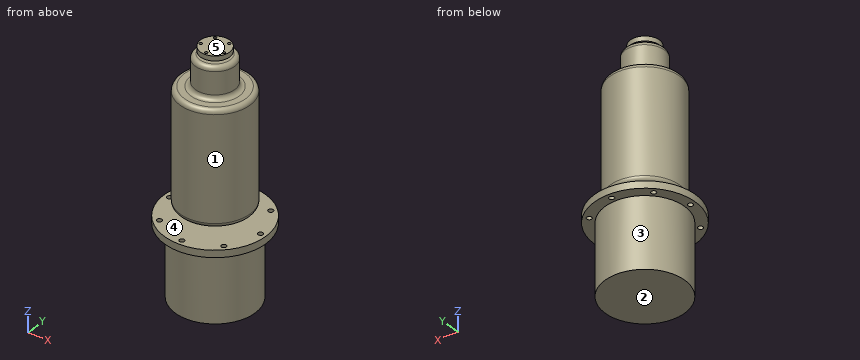
from build123d import *

# Parameters (mm, degrees)
SKETCH1_R          = 57.15
EXTRUDE1_DEPTH     = 4
SKETCH3_R          = 7.5
EXTRUDE2_DEPTH     = 12.166
SKETCH4_R          = 39.5
EXTRUDE3_DEPTH     = 127.24
SKETCH5_R          = 22.225
EXTRUDE4_DEPTH     = 35.083496
SKETCH6_R          = 9.525
EXTRUDE5_DEPTH     = 2.702052
SKETCH7_R          = 16.5
EXTRUDE6_DEPTH     = 5.3848
SKETCH8_R          = 1.6
CUT_EXTRUDE1_DEPTH = 5.3848
SKETCH10_R         = 2.79
CUT_EXTRUDE2_DEPTH = 8
SKETCH11_R         = 45
EXTRUDE7_DEPTH     = 79.4
FILLET1_R          = 5


with BuildPart() as part:
    # Sketch1 → Extrude1 (new body, symmetric)
    with BuildSketch(Plane.XY):
        Circle(SKETCH1_R)
    extrude(amount=EXTRUDE1_DEPTH, both=True)

    # Sketch3 → Extrude2 (add)
    with BuildSketch(Plane.XY.offset(4)):
        Circle(SKETCH3_R)
    extrude(amount=EXTRUDE2_DEPTH)

    # Sketch4 → Extrude3 (add)
    with BuildSketch(Plane.XY.offset(16.166)):
        Circle(SKETCH4_R)
    extrude(amount=EXTRUDE3_DEPTH)

    # Sketch5 → Extrude4 (add)
    with BuildSketch(Plane.XY.offset(143.406)):
        Circle(SKETCH5_R)
    extrude(amount=EXTRUDE4_DEPTH)

    # Sketch6 → Extrude5 (add)
    with BuildSketch(Plane.XY.offset(178.489496)):
        Circle(SKETCH6_R)
    extrude(amount=EXTRUDE5_DEPTH)

    # Sketch7 → Extrude6 (add)
    with BuildSketch(Plane.XY.offset(181.191548)):
        Circle(SKETCH7_R)
    extrude(amount=EXTRUDE6_DEPTH)

    # Sketch8 → Cut-Extrude1 (cut)
    with BuildSketch(Plane.XY.offset(186.576348)):
        with Locations((-7.935100906, 10.921729424)):
            Circle(SKETCH8_R)
        with Locations((7.935100906, 10.921729424)):
            Circle(SKETCH8_R)
        with Locations((12.83926297, -4.171729424)):
            Circle(SKETCH8_R)
        with Locations((0, -13.5)):
            Circle(SKETCH8_R)
        with Locations((-12.83926297, -4.171729424)):
            Circle(SKETCH8_R)
    extrude(amount=-CUT_EXTRUDE1_DEPTH, mode=Mode.SUBTRACT)

    # Sketch10 → Cut-Extrude2 (cut)
    with BuildSketch(Plane(origin=(0, 0, -4), x_dir=(-1, 0, 0), z_dir=(0, 0, -1))):
        with Locations((0, 50.8)):
            Circle(SKETCH10_R)
        with Locations((35.921024484, 35.921024484)):
            Circle(SKETCH10_R)
        with Locations((50.8, 0)):
            Circle(SKETCH10_R)
        with Locations((35.921024484, -35.921024484)):
            Circle(SKETCH10_R)
        with Locations((0, -50.8)):
            Circle(SKETCH10_R)
        with Locations((-35.921024484, -35.921024484)):
            Circle(SKETCH10_R)
        with Locations((-50.8, 0)):
            Circle(SKETCH10_R)
        with Locations((-35.921024484, 35.921024484)):
            Circle(SKETCH10_R)
    extrude(amount=-CUT_EXTRUDE2_DEPTH, mode=Mode.SUBTRACT)

    # Sketch11 → Extrude7 (add)
    with BuildSketch(Plane(origin=(0, 0, -4), x_dir=(-1, 0, 0), z_dir=(0, 0, -1))):
        with Locations(Location((0, 0, 0), (0, 0, 180))):  # turned: the seam where the file's is
            Circle(SKETCH11_R)
    extrude(amount=EXTRUDE7_DEPTH)

    # Fillet1
    fillet1_edges = [part.edges().sort_by_distance(p)[0] for p in [
        (-39.5, 0, 143.406),
        (-22.225, 0, 143.406),
        (-22.225, 0, 178.489496),
        (-39.5, 0, 16.166),
    ]]
    fillet(fillet1_edges, radius=FILLET1_R)


solid = part.part
The listing builds one solid part. Answer for the finished solid, in the listing's coordinates (mm). Face numbers are marked on the shaded views. A direction names the side the tool comes from. Round coordinates to 2 decimals unless told otherwise and drop trailing zeros. Write each loop counter-clockwise with the first axis right and the second up, starting at its lowest first coordinate (ties: lowest second). Pieces come first, ordered by that corner, then holes. Notation, with made-up numbers: (-34.5, 61) - (-27.5, 61) arc R23 cw to (-27.5, 74) - close; hole circle Ø11 at (-11.5, 84). An arc over 180 degrees is marked (long way). Use a Markdown table: item, result. Add a question column.
1. The part is cut by section A-A (x = 50.8). Write down the section's boundary in (y, z).
2. Flat-ended cylindrical pins translate along their axes: P1, Ø1, axis at x = 18, z = 27, coming from the -Y side; P2, Ø6, axis at x = 20, z = 95.5, coming from the +Y side; P3, Ø1, axis at x = 17, y = -43.5, coming from the +Z side; P4, Ø5, axis at x = 35.92, y = 35.92, coming from the -Z side. Find the tip coordinate at first contact, or state that the pin passes through.
3. A tool of negligible diameter and unlimited length cuts with its end or side. For the marked faces 1 and 2, from which of +Z, -Z, +X, -X, +Y, -Y can it reach the whole face along a straight path? Write none if from no direction.
4. The part is cut by section C-C (y = 0). Give the number of separate pieces and of enclosed holes in the cut face, and give its area (3 significant figures).
5. For a pull along Z with two mould halves and no side action, classify the marked faces 3, 4 and 5 as +Z half, -Z half, draft (parallel to the pull), parting line (faces both ways), or undercut.
6. Consider line 1 (Z direction, x = -14, y = 2); line 2 (Y direction, x = 0, z = 0.5); line 3 (Z direction, x = 31, y = 5.5). Determine where each line is inside the solid, lowest interval first.
Reported:
| question | item | result |
|---|---|---|
| 1 | outline | (-26.18, -4) - (-2.79, -4) - (-2.79, 4) - (-26.18, 4) - close; (2.79, -4) - (26.18, -4) - (26.18, 4) - (2.79, 4) - close |
| 2 | P1 | y = -35.41 |
| 2 | P2 | y = 35.65 |
| 2 | P3 | z = 4 |
| 2 | P4 | through |
| 3 | face 1 | +Z |
| 3 | face 2 | -Z, +X, -X, +Y, -Y |
| 4 | separate pieces | 3 |
| 4 | enclosed holes | 0 |
| 4 | area | 20,000 mm^2 |
| 5 | face 3 | draft |
| 5 | face 4 | undercut |
| 5 | face 5 | +Z half |
| 6 | line 1 | -83.4 to 4, 16.17 to 178.49, 181.19 to 186.58 |
| 6 | line 2 | -57.15 to -53.59, -48.01 to 48.01, 53.59 to 57.15 |
| 6 | line 3 | -83.4 to 4, 16.17 to 143.41 |
